Model file for the job. Use its own axes, mm. Coordinates: 2 decimals unless noted, no trailing zeros. Write item = value, one per line. Start each with the question number.
Q1. Cut at A-A, the plane z = 62.5. Give the number of separate pieces and of enclosed holes in the cut face, plus the area to 3 significant figures.
Q2. Flat gauge pin, fed straight in: pin 1 (3.5 mm diameter, centred on x = -42, z = 24, fed in from +Y). Where does the tip first touch, or does it go through?
Q3. Mould opens along Z. For faces 1 (the face through (-60.57, 1.61, -69)), 2 (the face through (62, 2, 1)), 3 (the face through (6.09, 1.57, 60.45)) say: +Z half, -Z half, draft (parallel to the pull), parting line (faces both ways), or undercut.
from build123d import *

# Parameters (mm, degrees)
SKETCH1_W           = 124
SKETCH1_H           = 141
SKETCH1_R           = 2.05
BOSS_EXTRUDE1_DEPTH = 3.175
FILLET1_R           = 5


with BuildPart() as part:
    # Sketch1 → Boss-Extrude1 (new body)
    with BuildSketch(Plane(origin=(0, 0, 0), x_dir=(1, 0, 0), z_dir=(0, 1, 0))):
        Rectangle(SKETCH1_W, SKETCH1_H)
        with Locations(Location((-58, -62.5, 0), (0, 0, 270))):
            Circle(SKETCH1_R, mode=Mode.SUBTRACT)
        with Locations(Location((-42, -62.5, 0), (0, 0, 270))):
            Circle(SKETCH1_R, mode=Mode.SUBTRACT)
        with Locations(Location((-26, -62.5, 0), (0, 0, 270))):
            Circle(SKETCH1_R, mode=Mode.SUBTRACT)
        with Locations(Location((-10, -62.5, 0), (0, 0, 270))):
            Circle(SKETCH1_R, mode=Mode.SUBTRACT)
        with Locations(Location((6, -62.5, 0), (0, 0, 270))):
            Circle(SKETCH1_R, mode=Mode.SUBTRACT)
        with Locations(Location((22, -62.5, 0), (0, 0, 270))):
            Circle(SKETCH1_R, mode=Mode.SUBTRACT)
        with Locations(Location((38, -62.5, 0), (0, 0, 270))):
            Circle(SKETCH1_R, mode=Mode.SUBTRACT)
        with Locations(Location((54, -62.5, 0), (0, 0, 270))):
            Circle(SKETCH1_R, mode=Mode.SUBTRACT)
        with Locations(Location((38, -40, 0), (0, 0, 270))):
            Circle(SKETCH1_R, mode=Mode.SUBTRACT)
        with Locations(Location((22, -40, 0), (0, 0, 270))):
            Circle(SKETCH1_R, mode=Mode.SUBTRACT)
        with Locations(Location((6, -40, 0), (0, 0, 270))):
            Circle(SKETCH1_R, mode=Mode.SUBTRACT)
        with Locations(Location((-10, -40, 0), (0, 0, 270))):
            Circle(SKETCH1_R, mode=Mode.SUBTRACT)
        with Locations(Location((-26, -40, 0), (0, 0, 270))):
            Circle(SKETCH1_R, mode=Mode.SUBTRACT)
        with Locations(Location((-42, -40, 0), (0, 0, 270))):
            Circle(SKETCH1_R, mode=Mode.SUBTRACT)
        with Locations(Location((-58, -40, 0), (0, 0, 270))):
            Circle(SKETCH1_R, mode=Mode.SUBTRACT)
        with Locations(Location((38, -24, 0), (0, 0, 270))):
            Circle(SKETCH1_R, mode=Mode.SUBTRACT)
        with Locations(Location((22, -24, 0), (0, 0, 270))):
            Circle(SKETCH1_R, mode=Mode.SUBTRACT)
        with Locations(Location((6, -24, 0), (0, 0, 270))):
            Circle(SKETCH1_R, mode=Mode.SUBTRACT)
        with Locations(Location((-10, -24, 0), (0, 0, 270))):
            Circle(SKETCH1_R, mode=Mode.SUBTRACT)
        with Locations(Location((-26, -24, 0), (0, 0, 270))):
            Circle(SKETCH1_R, mode=Mode.SUBTRACT)
        with Locations(Location((-42, -24, 0), (0, 0, 270))):
            Circle(SKETCH1_R, mode=Mode.SUBTRACT)
        with Locations(Location((-58, -24, 0), (0, 0, 270))):
            Circle(SKETCH1_R, mode=Mode.SUBTRACT)
        with Locations(Location((38, -8, 0), (0, 0, 270))):
            Circle(SKETCH1_R, mode=Mode.SUBTRACT)
        with Locations(Location((22, -8, 0), (0, 0, 270))):
            Circle(SKETCH1_R, mode=Mode.SUBTRACT)
        with Locations(Location((6, -8, 0), (0, 0, 270))):
            Circle(SKETCH1_R, mode=Mode.SUBTRACT)
        with Locations(Location((-10, -8, 0), (0, 0, 270))):
            Circle(SKETCH1_R, mode=Mode.SUBTRACT)
        with Locations(Location((-26, -8, 0), (0, 0, 270))):
            Circle(SKETCH1_R, mode=Mode.SUBTRACT)
        with Locations(Location((-42, -8, 0), (0, 0, 270))):
            Circle(SKETCH1_R, mode=Mode.SUBTRACT)
        with Locations(Location((-58, -8, 0), (0, 0, 270))):
            Circle(SKETCH1_R, mode=Mode.SUBTRACT)
        with Locations(Location((38, 8, 0), (0, 0, 270))):
            Circle(SKETCH1_R, mode=Mode.SUBTRACT)
        with Locations(Location((22, 8, 0), (0, 0, 270))):
            Circle(SKETCH1_R, mode=Mode.SUBTRACT)
        with Locations(Location((6, 8, 0), (0, 0, 270))):
            Circle(SKETCH1_R, mode=Mode.SUBTRACT)
        with Locations(Location((-10, 8, 0), (0, 0, 270))):
            Circle(SKETCH1_R, mode=Mode.SUBTRACT)
        with Locations(Location((-26, 8, 0), (0, 0, 270))):
            Circle(SKETCH1_R, mode=Mode.SUBTRACT)
        with Locations(Location((-42, 8, 0), (0, 0, 270))):
            Circle(SKETCH1_R, mode=Mode.SUBTRACT)
        with Locations(Location((-58, 8, 0), (0, 0, 270))):
            Circle(SKETCH1_R, mode=Mode.SUBTRACT)
        with Locations(Location((38, 24, 0), (0, 0, 270))):
            Circle(SKETCH1_R, mode=Mode.SUBTRACT)
        with Locations(Location((22, 24, 0), (0, 0, 270))):
            Circle(SKETCH1_R, mode=Mode.SUBTRACT)
        with Locations(Location((6, 24, 0), (0, 0, 270))):
            Circle(SKETCH1_R, mode=Mode.SUBTRACT)
        with Locations(Location((-10, 24, 0), (0, 0, 270))):
            Circle(SKETCH1_R, mode=Mode.SUBTRACT)
        with Locations(Location((-26, 24, 0), (0, 0, 270))):
            Circle(SKETCH1_R, mode=Mode.SUBTRACT)
        with Locations(Location((-42, 24, 0), (0, 0, 270))):
            Circle(SKETCH1_R, mode=Mode.SUBTRACT)
        with Locations(Location((-58, 24, 0), (0, 0, 270))):
            Circle(SKETCH1_R, mode=Mode.SUBTRACT)
        with Locations(Location((38, 40, 0), (0, 0, 270))):
            Circle(SKETCH1_R, mode=Mode.SUBTRACT)
        with Locations(Location((22, 40, 0), (0, 0, 270))):
            Circle(SKETCH1_R, mode=Mode.SUBTRACT)
        with Locations(Location((6, 40, 0), (0, 0, 270))):
            Circle(SKETCH1_R, mode=Mode.SUBTRACT)
        with Locations(Location((-10, 40, 0), (0, 0, 270))):
            Circle(SKETCH1_R, mode=Mode.SUBTRACT)
        with Locations(Location((-26, 40, 0), (0, 0, 270))):
            Circle(SKETCH1_R, mode=Mode.SUBTRACT)
        with Locations(Location((-42, 40, 0), (0, 0, 270))):
            Circle(SKETCH1_R, mode=Mode.SUBTRACT)
        with Locations(Location((-58, 40, 0), (0, 0, 270))):
            Circle(SKETCH1_R, mode=Mode.SUBTRACT)
        with Locations(Location((54, -40, 0), (0, 0, 270))):
            Circle(SKETCH1_R, mode=Mode.SUBTRACT)
        with Locations(Location((54, -24, 0), (0, 0, 270))):
            Circle(SKETCH1_R, mode=Mode.SUBTRACT)
        with Locations(Location((54, -8, 0), (0, 0, 270))):
            Circle(SKETCH1_R, mode=Mode.SUBTRACT)
        with Locations(Location((54, 8, 0), (0, 0, 270))):
            Circle(SKETCH1_R, mode=Mode.SUBTRACT)
        with Locations(Location((54, 24, 0), (0, 0, 270))):
            Circle(SKETCH1_R, mode=Mode.SUBTRACT)
        with Locations(Location((54, 40, 0), (0, 0, 270))):
            Circle(SKETCH1_R, mode=Mode.SUBTRACT)
        with Locations(Location((-58, 62.5, 0), (0, 0, 90))):
            Circle(SKETCH1_R, mode=Mode.SUBTRACT)
        with Locations(Location((-42, 62.5, 0), (0, 0, 90))):
            Circle(SKETCH1_R, mode=Mode.SUBTRACT)
        with Locations(Location((-26, 62.5, 0), (0, 0, 90))):
            Circle(SKETCH1_R, mode=Mode.SUBTRACT)
        with Locations(Location((-10, 62.5, 0), (0, 0, 90))):
            Circle(SKETCH1_R, mode=Mode.SUBTRACT)
        with Locations(Location((6, 62.5, 0), (0, 0, 90))):
            Circle(SKETCH1_R, mode=Mode.SUBTRACT)
        with Locations(Location((22, 62.5, 0), (0, 0, 90))):
            Circle(SKETCH1_R, mode=Mode.SUBTRACT)
        with Locations(Location((38, 62.5, 0), (0, 0, 90))):
            Circle(SKETCH1_R, mode=Mode.SUBTRACT)
        with Locations(Location((54, 62.5, 0), (0, 0, 90))):
            Circle(SKETCH1_R, mode=Mode.SUBTRACT)
    extrude(amount=BOSS_EXTRUDE1_DEPTH)

    # Fillet1
    fillet1_edges = [part.edges().sort_by_distance(p)[0] for p in [
        (-62, 1.5875, -70.5),
        (62, 1.5875, -70.5),
        (62, 1.5875, 70.5),
        (-62, 1.5875, 70.5),
    ]]
    fillet(fillet1_edges, radius=FILLET1_R)


solid = part.part
Here are the results:
q1.separate_pieces = 9
q1.enclosed_holes = 0
q1.area = 290 mm²
q2.pin_1 = through
q3.face_1 = -Z half
q3.face_2 = draft
q3.face_3 = undercut
